```python
from build123d import *

# Parameters (mm, degrees)
SKETCH_1_W           = 106
SKETCH_1_H           = 16
EXTRUDE_1_DEPTH      = 11
SKETCH_2_W           = 5
SKETCH_2_H           = 10
CUT_EXTRUDE_1_DEPTH  = 17
SKETCH_3_W           = 1
SKETCH_3_H           = 10
CUT_EXTRUDE_2_DEPTH  = 17
SKETCH_4_W           = 1
SKETCH_4_H           = 10
CUT_EXTRUDE_3_DEPTH  = 17
SKETCH_5_W           = 1
SKETCH_5_H           = 10
CUT_EXTRUDE_4_DEPTH  = 17
SKETCH_6_W           = 1
SKETCH_6_H           = 10
CUT_EXTRUDE_5_DEPTH  = 17
SKETCH_7_W           = 1
SKETCH_7_H           = 10
CUT_EXTRUDE_6_DEPTH  = 17
SKETCH_8_W           = 10.4
SKETCH_8_H           = 10.4
CUT_EXTRUDE_7_DEPTH  = 10
SKETCH_9_W           = 10.5
SKETCH_9_H           = 10.5
CUT_EXTRUDE_8_DEPTH  = 10
SKETCH_10_W          = 10.6
SKETCH_10_H          = 10.6
CUT_EXTRUDE_9_DEPTH  = 10
SKETCH_11_W          = 10.7
SKETCH_11_H          = 10.7
CUT_EXTRUDE_10_DEPTH = 10
SKETCH_12_W          = 10.8
SKETCH_12_H          = 10.8
CUT_EXTRUDE_11_DEPTH = 10
SKETCH_13_W          = 10.9
SKETCH_13_H          = 10.9
CUT_EXTRUDE_12_DEPTH = 10


with BuildPart() as part:
    # 草图1 → 凸台-拉伸1 (new body)
    with BuildSketch(Plane(origin=(0, 0, 0), x_dir=(-1, 0, 0), z_dir=(0, 0, -1))):
        with Locations((-53, -28)):
            Rectangle(SKETCH_1_W, SKETCH_1_H)
    extrude(amount=-EXTRUDE_1_DEPTH)

    # 草图2 → 切除-拉伸1 (cut, through all)
    with BuildSketch(Plane(origin=(0, -20, 0), x_dir=(-1, 0, 0), z_dir=(0, 1, 0))):
        with Locations((-103.5, 6)):
            Rectangle(SKETCH_2_W, SKETCH_2_H)
    extrude(amount=-CUT_EXTRUDE_1_DEPTH, mode=Mode.SUBTRACT)

    # 草图3 → 切除-拉伸2 (cut, through all)
    with BuildSketch(Plane(origin=(0, -20, 0), x_dir=(-1, 0, 0), z_dir=(0, 1, 0))):
        with Locations((-84.5, 6)):
            Rectangle(SKETCH_3_W, SKETCH_3_H)
    extrude(amount=-CUT_EXTRUDE_2_DEPTH, mode=Mode.SUBTRACT)

    # 草图4 → 切除-拉伸3 (cut, through all)
    with BuildSketch(Plane(origin=(0, -20, 0), x_dir=(-1, 0, 0), z_dir=(0, 1, 0))):
        with Locations((-67.5, 6)):
            Rectangle(SKETCH_4_W, SKETCH_4_H)
    extrude(amount=-CUT_EXTRUDE_3_DEPTH, mode=Mode.SUBTRACT)

    # 草图5 → 切除-拉伸4 (cut, through all)
    with BuildSketch(Plane(origin=(0, -20, 0), x_dir=(-1, 0, 0), z_dir=(0, 1, 0))):
        with Locations((-50.5, 6)):
            Rectangle(SKETCH_5_W, SKETCH_5_H)
    extrude(amount=-CUT_EXTRUDE_4_DEPTH, mode=Mode.SUBTRACT)

    # 草图6 → 切除-拉伸5 (cut, through all)
    with BuildSketch(Plane(origin=(0, -20, 0), x_dir=(-1, 0, 0), z_dir=(0, 1, 0))):
        with Locations((-33.5, 6)):
            Rectangle(SKETCH_6_W, SKETCH_6_H)
    extrude(amount=-CUT_EXTRUDE_5_DEPTH, mode=Mode.SUBTRACT)

    # 草图7 → 切除-拉伸6 (cut, through all)
    with BuildSketch(Plane(origin=(0, -20, 0), x_dir=(-1, 0, 0), z_dir=(0, 1, 0))):
        with Locations((-16.5, 6)):
            Rectangle(SKETCH_7_W, SKETCH_7_H)
    extrude(amount=-CUT_EXTRUDE_6_DEPTH, mode=Mode.SUBTRACT)

    # 草图8 → 切除-拉伸7 (cut)
    with BuildSketch(Plane.XY.offset(11)):
        with Locations((8, -28)):
            Rectangle(SKETCH_8_W, SKETCH_8_H)
    extrude(amount=-CUT_EXTRUDE_7_DEPTH, mode=Mode.SUBTRACT)

    # 草图9 → 切除-拉伸8 (cut)
    with BuildSketch(Plane.XY.offset(11)):
        with Locations((25, -28)):
            Rectangle(SKETCH_9_W, SKETCH_9_H)
    extrude(amount=-CUT_EXTRUDE_8_DEPTH, mode=Mode.SUBTRACT)

    # 草图10 → 切除-拉伸9 (cut)
    with BuildSketch(Plane.XY.offset(11)):
        with Locations((42, -28)):
            Rectangle(SKETCH_10_W, SKETCH_10_H)
    extrude(amount=-CUT_EXTRUDE_9_DEPTH, mode=Mode.SUBTRACT)

    # 草图11 → 切除-拉伸10 (cut)
    with BuildSketch(Plane.XY.offset(11)):
        with Locations((59, -28)):
            Rectangle(SKETCH_11_W, SKETCH_11_H)
    extrude(amount=-CUT_EXTRUDE_10_DEPTH, mode=Mode.SUBTRACT)

    # 草图12 → 切除-拉伸11 (cut)
    with BuildSketch(Plane.XY.offset(11)):
        with Locations((76, -28)):
            Rectangle(SKETCH_12_W, SKETCH_12_H)
    extrude(amount=-CUT_EXTRUDE_11_DEPTH, mode=Mode.SUBTRACT)

    # 草图13 → 切除-拉伸12 (cut)
    with BuildSketch(Plane.XY.offset(11)):
        with Locations((93, -28)):
            Rectangle(SKETCH_13_W, SKETCH_13_H)
    extrude(amount=-CUT_EXTRUDE_12_DEPTH, mode=Mode.SUBTRACT)


solid = part.part
```
Read the model definition and answer for the solid it produces. Units are mm, in the model's axes. A direction names the side the tool comes from. Round coordinates to 2 decimals unless told otherwise and drop trailing zeros. Write each loop counter-clockwise with the first axis right and the second up, starting at its lowest first coordinate (ties: lowest second). Pieces come first, ordered by that corner, then holes. Notation, with made-up numbers: M -8,7.25 L 27,7.25 A13 cw 27,24.25 Z; hole C -0.5,14.5 d1. An arc over 180 degrees is marked long. One line per item, written item: value.
Q1. Find section D-D on x = 38. Write down the section's boundary in (y, z), plus the area to 3 significant figures.
Data:
outline: M -36,0 L -20,0 L -20,11 L -22.7,11 L -22.7,1 L -33.3,1 L -33.3,11 L -36,11 Z
area: 70.0 mm2
Q2. Flat-ended cylindrical pins translate along their axes: pin 1 Ø5 at (y, z) = (-26, 6.5) entering from +X; pin 2 Ø0.5 at (x, y) = (16.5, -24) entering from +Z. Find the tip coordinate at first contact, or state that the pin passes through.
Data:
pin 1: x = 101
pin 2: z = 1
Q3. For a pull along X with two mould halves and no side action, classify faces 4 (the flat face through (104, -28, 1)), 5 (the flat face through (42, -33.3, 6)), 6 (the flat face through (0, -28, 5)) as +X half, -X half, draft (parallel to the pull), parting line (faces both ways), or undercut.
Data:
face 4: draft
face 5: undercut
face 6: -X half
Q4. Straight lines are drawn through the part: line 1 (X direction, y = -35, z = 4.5); line 2 (Y direction, x = 75, z = 6.75); line 3 (Y direction, x = 13, z = 9). For each, find the intervals that lie inside material, in ascending order. Write a range as [from, to].
Data:
line 1: [0, 16], [17, 33], [34, 50], [51, 67], [68, 84], [85, 101]
line 2: [-36, -33.4], [-22.6, -20]
line 3: [-36, -33.2], [-22.8, -20]
Q5. Which of the six approach directions +Z, -Z, +X, -X, +Y, -Y give full straight-line access (tool end or side, diameter ignored) to faces 1 (the flat face through (54, -20, 5)), 2 (the flat face through (84, -28, 6)), 3 (the flat face through (93, -33.45, 6))?
Data:
face 1: +Z, -Z, +X, -X, +Y
face 2: +Z, +Y, -Y
face 3: +Z
Q6. Find section C-C on y = -34.75. Write down the section's boundary in (x, z).
Data:
outline: M 0,0 L 106,0 L 106,1 L 101,1 L 101,11 L 85,11 L 85,1 L 84,1 L 84,11 L 68,11 L 68,1 L 67,1 L 67,11 L 51,11 L 51,1 L 50,1 L 50,11 L 34,11 L 34,1 L 33,1 L 33,11 L 17,11 L 17,1 L 16,1 L 16,11 L 0,11 Z
Q7. Find section B-B on x = 91. Write down the section's boundary in (y, z), plus the area to 3 significant figures.
Data:
outline: M -36,0 L -20,0 L -20,11 L -22.55,11 L -22.55,1 L -33.45,1 L -33.45,11 L -36,11 Z
area: 67.0 mm2
Q8. Find section A-A on z = 3.75. Count the separate pieces of the cut face and the enclosed holes in it, plus the area to 3 significant figures.
Data:
separate pieces: 6
enclosed holes: 6
area: 855 mm2
